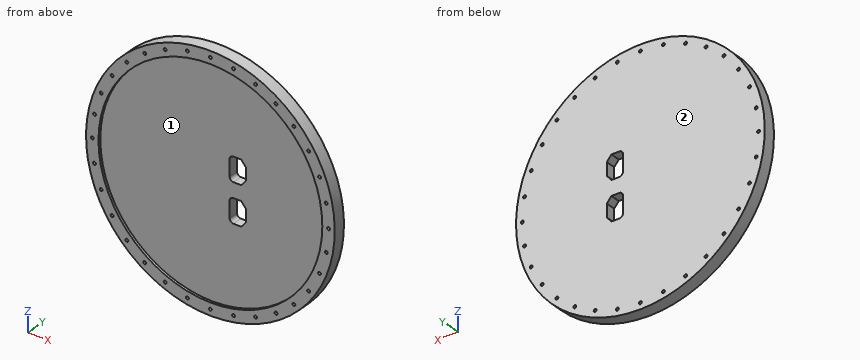
```python
from build123d import *

# Parameters (mm, degrees)
CUT_EXTRUDE2_DEPTH = 1.2
SKETCH4_R          = 0.175
CUT_EXTRUDE3_DEPTH = 1.5
CIRPATTERN1_COUNT  = 32
SCALE1_SCALE       = 5


with BuildPart() as part:
    # Sketch2 → Revolve1 (revolve)
    with BuildSketch(Plane.XY, mode=Mode.PRIVATE) as revolve1_sk:
        Polygon((13.5, 0), (13.5, 0.3), (0, 0.3), (0, 1.5), (15, 1.5), (15, 0), align=None)
    revolve(revolve1_sk.sketch.rotate(Axis((0, 0, 0), (0, 1, 0)), 90), axis=Axis((0, 0, 0), (0, 1, 0)))

    # Sketch3 → Cut-Extrude2 (cut)
    with BuildSketch(Plane(origin=(0, 1.5, 0), x_dir=(1, 0, 0), z_dir=(0, 1, 0))):
        with BuildLine():
            Line((2.1, -3.35), (2.1, -1.35))
            ThreePointArc((2.1, -1.35), (2.231801948, -1.031801948), (2.55, -0.9))
            Line((2.55, -0.9), (3.496837495, -0.9))
            Line((3.496837495, -0.9), (4.05, -1.563795006))
            Line((4.05, -1.563795006), (4.05, -3.136204994))
            Line((4.05, -3.136204994), (3.496837495, -3.8))
            Line((3.496837495, -3.8), (2.55, -3.8))
            ThreePointArc((2.55, -3.8), (2.231801948, -3.668198052), (2.1, -3.35))
        make_face()
        with BuildLine():
            Line((3.496837495, 3.8), (2.55, 3.8))
            ThreePointArc((2.55, 3.8), (2.231801948, 3.668198052), (2.1, 3.35))
            Line((2.1, 3.35), (2.1, 1.35))
            ThreePointArc((2.1, 1.35), (2.231801948, 1.031801948), (2.55, 0.9))
            Line((2.55, 0.9), (3.496837495, 0.9))
            Line((3.496837495, 0.9), (4.05, 1.563795006))
            Line((4.05, 1.563795006), (4.05, 3.136204994))
            Line((4.05, 3.136204994), (3.496837495, 3.8))
        make_face()
    extrude(amount=-CUT_EXTRUDE2_DEPTH, mode=Mode.SUBTRACT)

    # Sketch4 → Cut-Extrude3 (cut)
    with BuildSketch(Plane(origin=(0, 1.5, 0), x_dir=(1, 0, 0), z_dir=(0, 1, 0))):
        with Locations(Location((14.25, 0, 0), (0, 0, 270))):
            Circle(SKETCH4_R)
    cut_extrude3 = extrude(amount=-CUT_EXTRUDE3_DEPTH, mode=Mode.SUBTRACT)

    # CirPattern1: Cut-Extrude3 ×32 about axis
    cirpattern1_axis = Axis((0, 0, 0), (0, 1, 0))
    for i in range(1, CIRPATTERN1_COUNT):
        add(cut_extrude3.rotate(cirpattern1_axis, i * 360 / CIRPATTERN1_COUNT), mode=Mode.SUBTRACT)


with BuildPart() as part_1:
    # Scale1: scaled about (-0.043455852, 0.866118001, 0)
    add(part.part.scale(SCALE1_SCALE).moved(Location((0.173823408, -3.464472004, 0))))


solid = part_1.part
```
Read the model definition and answer for the solid it produces. Units are mm, in the model's axes. Face numbers are marked on the shaded views. Give positions to 0.01 mm unless a question says otherwise; leave off trailing zeros. Loops run counter-clockwise (first coordinate to the right, second up) from the corner with the lowest first, then second, coordinate; pieces in that order, holes last.
Item 1: The part is cut by section A-A (x = 30.5). Write down the section's boundary in (y, z).
Item 2: The part is cut by section B-B (z = 45). Write down the section's boundary in (x, y), and give its area (3 significant figures).
Item 3: Each of these flat-tipped pins is pushed along its axis until it touches: pin 1 Ø2.5 at (x, y) = (16, 1.5) entering from -Z; pin 2 Ø2 at (x, y) = (-36, 2.5) entering from -Z; pin 3 Ø1.5 at (y, z) = (2.5, -16) entering from -X. Where does it stop, or does it pass through?
Item 4: The part is cut by section C-C (y = 2.5). Give the number of separate pieces and of enclosed holes in the cut face, and give its area (3 significant figures).
Item 5: Find the intervals of material crossed by line 1 along X through (y, z) = (1.25, -66); line 2 along X through (y, z) = (0.5, 50); line 3 along X through (y, z) = (-2.5, -60), in increasing order.
Item 6: The mould has two halves that part along X. Classify the marked faces 1 and 2: released by +X, released by -X, zero draft, split by the parting line, or undercut.
Taken from the geometry:
1. outline: (-3.46, -68.6) - (4.04, -68.6) - (4.04, 68.6) - (-3.46, 68.6) - (-3.46, 60.3) - (-1.96, 60.3) - (-1.96, -60.3) - (-3.46, -60.3) - close
2. outline: (-59.83, -3.46) - (-50.14, -3.46) - (-50.14, -1.96) - (50.49, -1.96) - (50.49, -3.46) - (60.17, -3.46) - (60.17, 4.04) - (-59.83, 4.04) - close
2. area: 749 mm2
3. pin 1: stops at z = -73.57
3. pin 2: stops at z = -66.24
3. pin 3: stops at x = -73.26
4. separate pieces: 1
4. enclosed holes: 34
4. area: 17,300 mm2
5. line 1: x = -35.45 to -27.95, -26.23 to 26.58, 28.3 to 35.8
5. line 2: x = -55.73 to -51, -49.42 to 49.77, 51.34 to 56.08
5. line 3: x = -44.83 to -39.85, -38.97 to -30.75, 31.1 to 39.32, 40.2 to 45.17
6. face 1: undercut
6. face 2: zero draft
